from build123d import *

# Parameters (mm, degrees)
COQUE1_T = -2


with BuildPart() as part:
    # Esquisse2 → Révolution1 (revolve)
    with BuildSketch(Plane.XY, mode=Mode.PRIVATE) as r_volution1_sk:
        Polygon((-393.705721225, 604.708824353), (-370.2870475, 595.9586403), (-419.288078193, 464.814067439), (-442.706751918, 473.564251491), (-439.55668566, 481.994974032), (-429.864663683, 500.791641556), (-401.864074716, 575.731397477), (-396.855787484, 596.278101812), align=None)
    revolve(r_volution1_sk.sketch.rotate(Axis((-437.599068934, 415.807199106, 0), (0.350007362, 0.936746949, 0)), 180), axis=Axis((-437.599068934, 415.807199106, 0), (0.350007362, 0.936746949, 0)))  # turned: the seam where the file's is

    # Coque1
    coque1_openings = [part.faces().sort_by_distance(p)[0] for p in [
        (-370.2870475, 595.9586403, 0),
        (-419.288078193, 464.814067439, 0),
    ]]
    offset(amount=COQUE1_T, openings=coque1_openings, kind=Kind.INTERSECTION)


solid = part.part
Design review of the part built by this model. Coordinates are the model's own, in mm. Coordinates: 2 decimals unless noted, no trailing zeros. Use one line per item in the form item = value.
Q1. The part is to be moulded in two halves that separate along Z. For faces 1 (the conical face through (-426.45, 490.83, -14.5)), 2 (the flat face through (-349.58, 588.22, 7.29)), 3 (the conical face through (-391.3, 477.82, 8.98)), say which applies: +Z half, -Z half, draft (parallel to the pull), parting line (faces both ways), or undercut.
Taken from the geometry:
face_1 = undercut
face_2 = draft
face_3 = parting line
Q2. Insertion check: pin 1 Ø3 at (x, z) = (-362.5, 20) entering from +Y; pin 2 Ø10 at (x, y) = (-381.5, 538.5) entering from -Z; pin 3 Ø10 at (y, z) = (471.5, -5.5) entering from +X. Each pin has a flat end and moves straight along its axis. Give the tip position at first contact, or say it passes through.
Taken from the geometry:
pin_1 = 593.09
pin_2 = -22.02
pin_3 = -390.15
Q3. For probe 1 along X at (y, z) = (537.5, -3); probe 2 along Z at (x, y) = (-359, 582); probe 3 along X at (y, z) = (544, 5.5), list the stretches that pass through material, from the lowest coordinate up.
Taken from the geometry:
probe_1 = -415.93 to -413.78, -370.48 to -368.32
probe_2 = -19.63 to -16.99, 16.99 to 19.63
probe_3 = -412.99 to -410.78, -368.62 to -366.41
